Answer from the drawing. Dimensions are ordinates in mm from the lowest x, y and z of the part. A direction names the side the tool comes from. Give positions to 0.01 mm unless a question says otherwise; leave off trailing zeros. Loops run counter-clockwise (first coordinate to the right, second up) from the corner with the lowest first, then second, coordinate; pieces in that order, holes last. Notation, with made-up numbers: (-39, -21.5) -> (-18, -21.5) arc R15 ccw to (-18, -4.5) -> close; hole circle Ø5 at (13.25, 17.25). An arc over 180 degrees is marked (long way). Return JSON: item names as keys, results as strings. Group by question number.
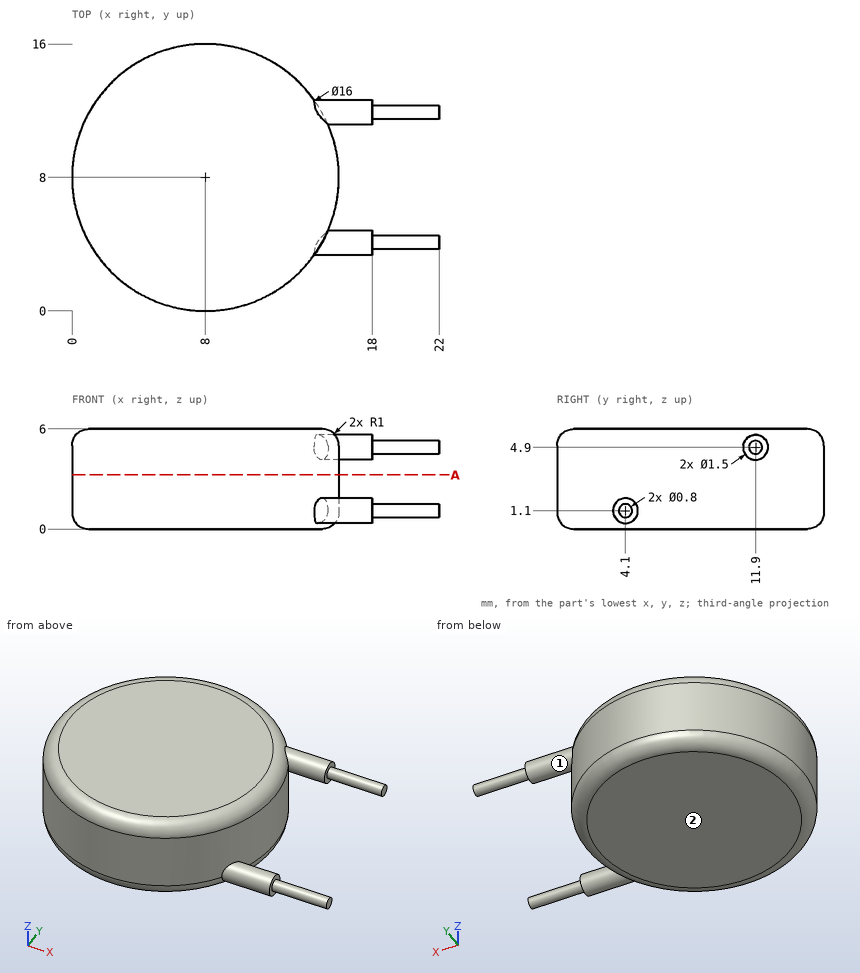
1. Which of the six approach directions +Z, -Z, +X, -X, +Y, -Y give full straight-line access (tool end or side, diameter ignored) to the marked faces 1 and 2?
2. Straight lines are drawn through the part: line 1 (X direction, y = 7.75, z = 5.5); line 2 (Y direction, x = 20.5, z = 1); line 3 (Y direction, x = 12, z = 0.75). For each, find the intervals that lie inside material, in ascending order. Write a range as from..to.
3. Flat-ended cylindrical pins translate along their axes: pin 1 Ø1 at (y, z) = (12, 3) entering from +X; pin 2 Ø1.5 at (x, y) = (16.5, 11.5) entering from -Z; pin 3 Ø3 at (x, z) = (4, 5.5) entering from -Y. Find the tip coordinate at first contact, or state that the pin passes through.
4. Section A-A on z = 3.25 is taken. Determine the outline of the cut face in (x, y), then the cut area to 3 significant figures.
Completed:
{
 "1": {"face 1": "+X", "face 2": "-Z, +X, -X, +Y, -Y"},
 "2": {"line 1": "x = 0.14..15.86", "line 2": "y = 3.71..4.49", "line 3": "y = 1.11..14.89"},
 "3": {"pin 1": "stops at x = 15.19", "pin 2": "stops at z = 4.15", "pin 3": "stops at y = 0.42"},
 "4": {"outline": "circle Ø16 at (8, 8)", "area": "201 mm²"}
}
